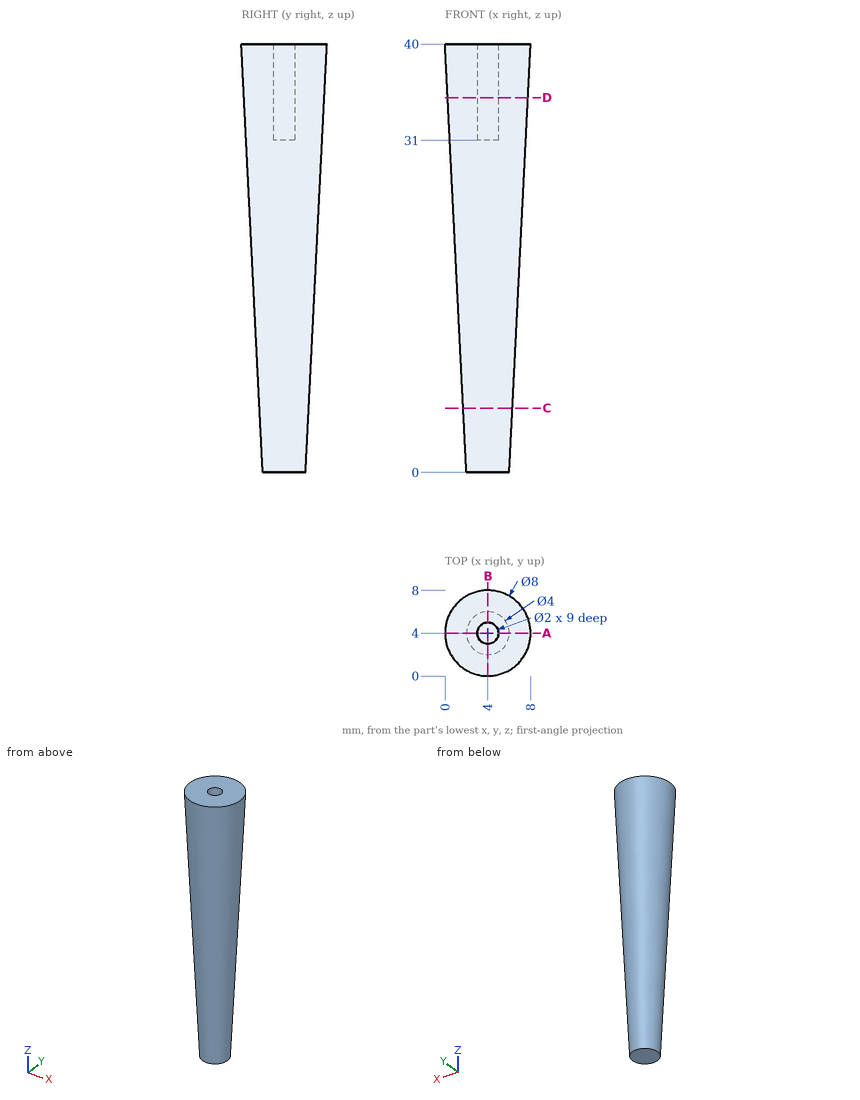
Verification items for this drawing (mm, ordinates from the low corner). Coordinates: 2 decimals unless noted, no trailing zeros. Order: outer loops, then holes, each group sorted by start corner. A loop starts at its lowest first (then second) coordinate and runs counter-clockwise, first axis right, second up.
Q1. Depth check by flat-ended pin: pin 1 Ø1 at (x, z) = (6.5, 34.5) entering from -Y; pin 2 Ø1.5 at (x, z) = (2.5, 7.5) entering from +Y; pin 3 Ø2 at (x, z) = (7, 9.5) entering from +Y. Enter the tip coordinate at first touch or a pass-through.
Reply:
pin 1: stops at y = 0.86
pin 2: stops at y = 6.26
pin 3: stops at y = 5.46
Q2. Sectioned sample at C-C on z = 6. Record the cut outline in (x, y).
Reply:
outline: circle Ø4.6 at (4, 4)
Q3. Thickness scan on probe 1 along X at (y, z) = (4, 37.25); probe 2 along Y at (x, z) = (4, 37.5) (3 decimals); probe 3 along Y at (x, z) = (4, 34). Record the ranges inside material, lowest first.
Reply:
probe 1: x = 0.14 to 3, 5 to 7.86
probe 2: y = 0.125 to 3, 5 to 7.875
probe 3: y = 0.3 to 3, 5 to 7.7
Q4. Sectioned sample at D-D on z = 35. Record the cut outline in (x, y).
Reply:
outline: circle Ø7.5 at (4, 4); hole circle Ø2 at (4, 4)
Q5. Sectioned sample at A-A on y = 4. Record the cut outline in (x, z).
Reply:
outline: (0, 40) - (2, 0) - (6, 0) - (8, 40) - (5, 40) - (5, 31) - (3, 31) - (3, 40) - close
